Check sheet for the drawn part. Datum: minimum x, y, z corner. Units: mm. Coordinates: 2 decimals unless noted, no trailing zeros. Order: outer loops, then holes, each group sorted by start corner. A loop starts at its lowest first (then second) coordinate and runs counter-clockwise, first axis right, second up.
Q1. Cross-section at B-B, the plane z = 25. Record the boundary of the cut face in (x, y), and give its area (3 significant figures).
Q2. Thickness scan on line 1 (Z direction, x = 25, y = 1.3); line 2 (Z direction, x = 48, y = 1.4); line 3 (X direction, y = 0.6, z = 25). Record the ranges inside material, lowest first.
Q3. Cross-section at A-A, the plane x = 25. Record the boundary of the cut face in (y, z), and give its area (3 significant figures).
Q4. Depth check by flat-ended pin: P1, Ø5, axis at x = 25, z = 25, coming from the -Y side; P2, Ø1.5, axis at y = 1.5, z = 5, coming from the +X side; P3, Ø0.9, axis at x = 2, y = 2, coming from the -Z side; P4, Ø6, axis at x = 40, z = 19, coming from the -Y side. Enter the tip coordinate at first touch or a pass-through.
Q5. Cross-section at C-C, the plane y = 0.6. Record the boundary of the cut face in (x, z), and give its area (3 significant figures).
Q6. Cross-section at D-D, the plane x = 31. Record the boundary of the cut face in (y, z).
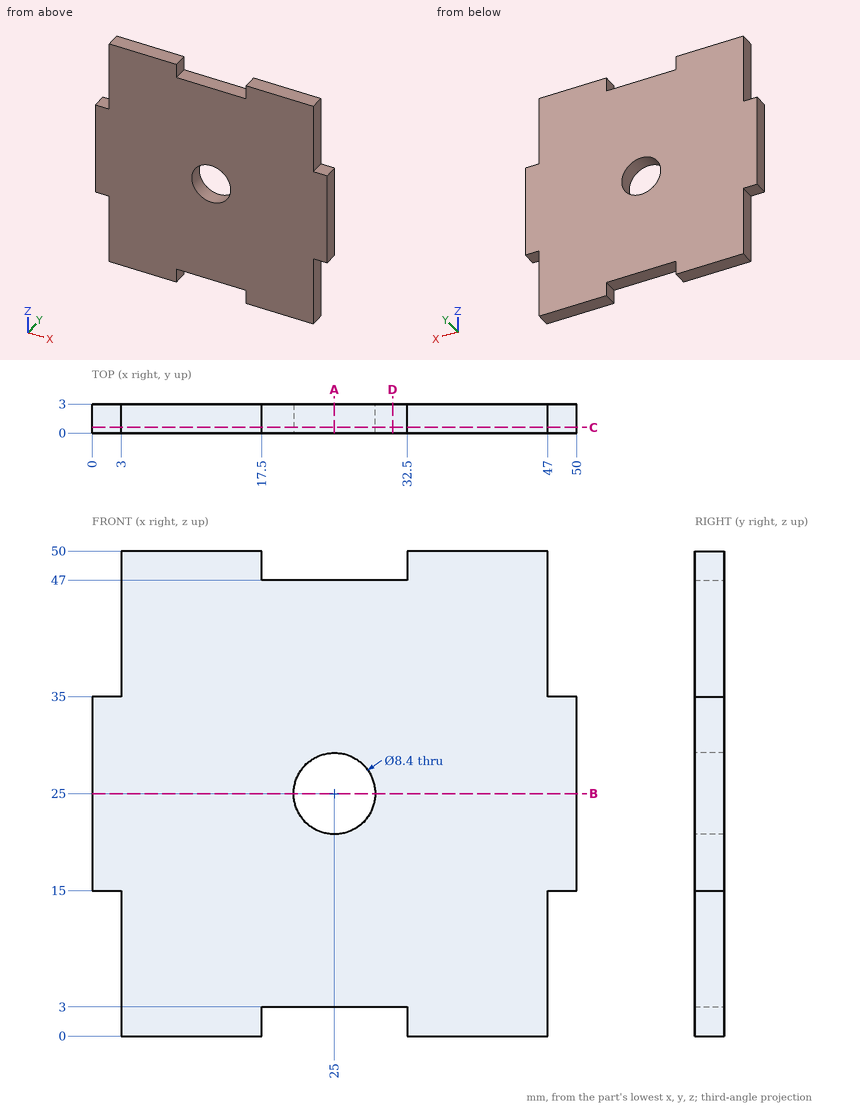
Check values:
1. outline: (0, 0) - (20.8, 0) - (20.8, 3) - (0, 3) - close; (29.2, 0) - (50, 0) - (50, 3) - (29.2, 3) - close
1. area: 125 mm2
2. line 1: z = 3 to 20.8, 29.2 to 47
2. line 2: z = 15 to 35
2. line 3: x = 0 to 20.8, 29.2 to 50
3. outline: (0, 3) - (3, 3) - (3, 20.8) - (0, 20.8) - close; (0, 29.2) - (3, 29.2) - (3, 47) - (0, 47) - close
3. area: 107 mm2
4. P1: passes through
4. P2: stops at x = 47
4. P3: stops at z = 15
4. P4: stops at y = 0
5. outline: (0, 15) - (3, 15) - (3, 0) - (17.5, 0) - (17.5, 3) - (32.5, 3) - (32.5, 0) - (47, 0) - (47, 15) - (50, 15) - (50, 35) - (47, 35) - (47, 50) - (32.5, 50) - (32.5, 47) - (17.5, 47) - (17.5, 50) - (3, 50) - (3, 35) - (0, 35) - close; hole circle Ø8.4 at (25, 25)
5. area: 2,170 mm2
6. outline: (0, 3) - (3, 3) - (3, 47) - (0, 47) - close
